Source: CAD feature listing. Evaluate the final solid. Frame: model axes, mm. Give positions to 0.01 mm unless a question says otherwise; leave off trailing zeros. Order: outer loops, then holes, each group sorted by start corner. A loop starts at its lowest first (then second) coordinate and runs counter-clockwise, first axis right, second up. Notation, with made-up numbers: M -32,65 L -3,65 A27 cw -3,96 Z; hole C 65.25,66 d3. An arc over 180 degrees is marked long. Answer as a JSON object with one key per item and string values. Group by question number.
1. Material intervals for L1, parallel to Y at x = -0.75, z = -196.5; L2, parallel to Y at x = -16, z = -130.5 (3 decimals); L3, parallel to X at y = 21, z = -128, sorted ascending. Write a range as [from, to].
2. Pin query (flat end, axial travel): P1, Ø12, axis at y = 13.5, z = -298, coming from the -X side; P2, Ø10.5, axis at y = 27, z = -148, coming from the +X side; P3, Ø4, axis at x = -3, y = 6.5, coming from the +Z side; P4, Ø6, axis at y = 5.5, z = -215.5, coming from the -X side. Return the tip coordinate at first contact, or that it passes through.
3. Section query B-B (y = 27.5). Output: boundary loops of the cut face in (x, z).
4. Section query A-A (z = -340.5). Output: boundary loops of the cut face in (x, y) (1 decimal).
from build123d import *

# Parameters (mm, degrees)
EXTRUDE_THIN1_DEPTH = 381
FILLET1_R           = 1.27


with BuildPart() as part:
    # Sketch1 → Extrude-Thin1 (new body)
    with BuildSketch(Plane.XY):
        with BuildLine():
            Line((0, 0), (-6.35, 0))
            ThreePointArc((-6.35, 0), (-7.150715566, 4.970497036), (-9.471846695, 9.438084357))
            Line((-9.471846695, 9.438084357), (-11.959403305, 12.786915643))
            ThreePointArc((-11.959403305, 12.786915643), (-14.280534434, 17.254502964), (-15.08125, 22.225))
            Line((-15.08125, 22.225), (-17.4625, 22.225))
            Line((-17.4625, 22.225), (-17.4625, 38.1))
            Line((-17.4625, 38.1), (0, 38.1))
            Line((0, 38.1), (0, 36.83))
            Line((0, 36.83), (-16.1925, 36.83))
            Line((-16.1925, 36.83), (-16.1925, 23.495))
            Line((-16.1925, 23.495), (-13.75574743, 23.495))
            ThreePointArc((-13.75574743, 23.495), (-13.261207377, 18.261141502), (-10.939897249, 13.544218358))
            Line((-10.939897249, 13.544218358), (-8.45234064, 10.195387073))
            ThreePointArc((-8.45234064, 10.195387073), (-6.155730596, 5.968907892), (-5.127232377, 1.27))
            Line((-5.127232377, 1.27), (0, 1.27))
            Line((0, 1.27), (0, 0))
        make_face()
    extrude(amount=-EXTRUDE_THIN1_DEPTH)

    # Fillet1
    fillet1_edges = [part.edges().sort_by_distance(p)[0] for p in [
        (-13.75574743, 23.495, -190.5),
        (-6.35, 0, -190.5),
        (-17.4625, 22.225, -190.5),
        (-17.4625, 38.1, -190.5),
    ]]
    fillet(fillet1_edges, radius=FILLET1_R)


solid = part.part
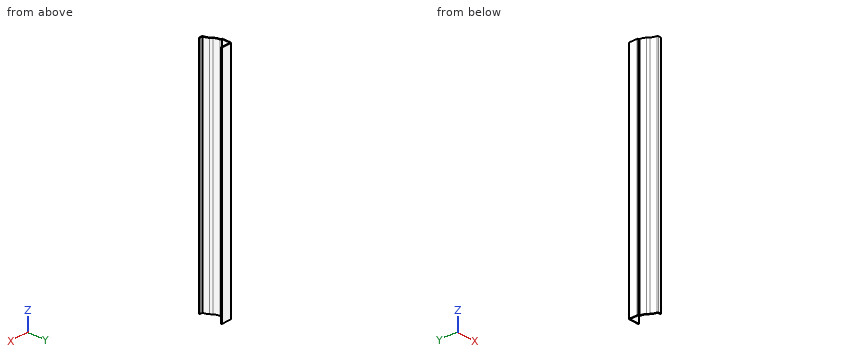
Answer sheet:
{
 "1": {"L1": "[0, 1.27], [36.83, 38.1]", "L2": "[22.225, 23.495], [36.83, 38.1]", "L3": "[-15.03, -13.76]"},
 "2": {"P1": "x = -14.84", "P2": "x = -13.8", "P3": "through", "P4": "x = -8.83"},
 "3": {"outline": "M -17.46,-381 L -16.19,-381 L -16.19,0 L -17.46,0 Z"},
 "4": {"outline": "M -17.5,23.5 A1.3 ccw -16.2,22.2 L -15.1,22.2 A15.8 ccw -12,12.8 L -9.5,9.4 A15.8 cw -6.4,1.2 A1.3 ccw -5.1,0 L 0,0 L 0,1.3 L -5.1,1.3 A17.1 ccw -8.5,10.2 L -10.9,13.5 A14.6 cw -13.8,22.2 A1.3 ccw -15.1,23.5 L -16.2,23.5 L -16.2,36.8 L 0,36.8 L 0,38.1 L -16.2,38.1 A1.3 ccw -17.5,36.8 Z"}
}
